Part print with two shaded views. Sizes in mm from the minimum x, y, z corner. A direction names the side the tool comes from. Round coordinates to 2 decimals unless told otherwise and drop trailing zeros. Loops run counter-clockwise (first coordinate to the right, second up) from the corner with the lowest first, then second, coordinate; pieces in that order, holes last. Notation, with made-up numbers: (55, 37) -> (96, 37) arc R28 ccw to (96, 62) -> close; hole circle Ø6 at (36.25, 53). An arc over 180 degrees is marked (long way). Answer as a JSON object with one key per item and string values. Group by question number.
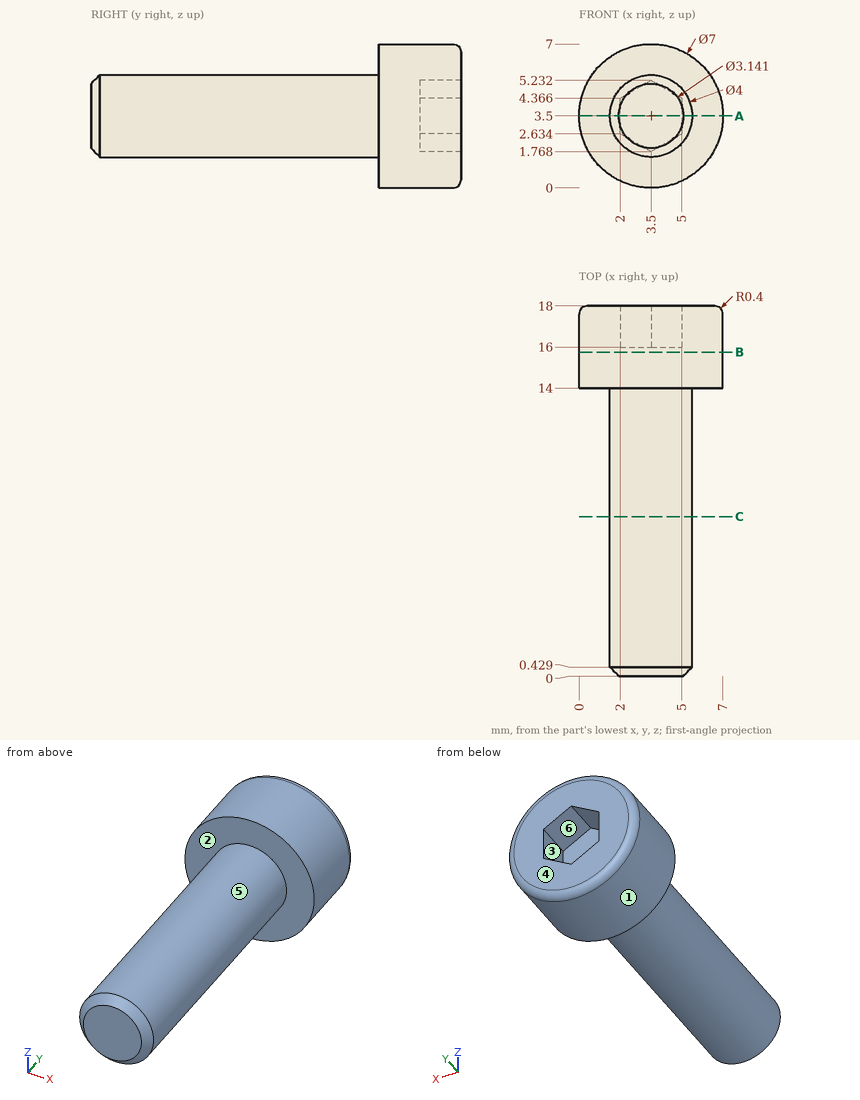
Item 1: Band-saw the part on C-C, the plane y = 7.75. List the corners of the cut face in (x, z).
Item 2: Which spindle directions (+Z, -Z, +X, -X, +Y, -Y) get a long thin tool onto all of the face, cutting with end or side? Do the marked faces 1 and 2. Say none if no direction does.
Item 3: Two-plate mould, pull along X, no slides. Class the marked faces 3, 4, 5 and 6: pulls with the +X half, pulls with the -X half, needs draft (parallel to the pull), parting line crosses it, or undercut.
Item 4: Band-saw the part on A-A, the plane z = 3.5. List the corners of the cut face in (x, y).
Item 5: Drill centre lines: line 1 (Y direction, x = 4, z = 4); line 2 (Y direction, x = 6, z = 4); line 3 (Z direction, x = 3.5, y = 8.5). Where is each one in solid material? Low to high.
Item 6: Drop flat-ended pins along their axis: pin 1 Ø1.5 at (x, z) = (4, 3) entering from +Y; pin 2 Ø1 at (x, y) = (5.5, 13) entering from -Z (1 decimal); pin 3 Ø4 at (y, z) = (6, 1.5) entering from -X. Give the stop position or say it passes through.
Item 7: Band-saw the part on B-B, the plane y = 15.75. List the corners of the cut face in (x, z).
Entries:
{
 "1": {"outline": "circle Ø4 at (3.5, 3.5)"},
 "2": {"face 1": "+Y, -Y", "face 2": "-Y"},
 "3": {"face 3": "undercut", "face 4": "needs draft", "face 5": "parting line crosses it", "face 6": "undercut"},
 "4": {"outline": "(0, 14) -> (1.5, 14) -> (1.5, 0.43) -> (1.93, 0) -> (5.07, 0) -> (5.5, 0.43) -> (5.5, 14) -> (7, 14) -> (7, 17.6) arc R0.4 ccw to (6.6, 18) -> (5, 18) -> (5, 16) -> (2, 16) -> (2, 18) -> (0.4, 18) arc R0.4 ccw to (0, 17.6) -> close"},
 "5": {"line 1": "0 to 16", "line 2": "14 to 18", "line 3": "1.5 to 5.5"},
 "6": {"pin 1": "y = 16", "pin 2": "z = 2.2", "pin 3": "x = 1.5"},
 "7": {"outline": "circle Ø7 at (3.5, 3.5)"}
}
